Read the model definition and answer for the solid it produces. Units are mm, in the model's axes. A direction names the side the tool comes from. Coordinates: 2 decimals unless noted, no trailing zeros. Loops run counter-clockwise (first coordinate to the right, second up) from the corner with the lowest first, then second, coordinate; pieces in that order, holes last. Notation, with made-up numbers: (43.25, 88) -> (57.25, 88) arc R20 ccw to (57.25, 95) -> close; hole circle Ø8 at (74.25, 23). An arc over 180 degrees is marked (long way). Answer as a JSON object with one key per item and string values. Group by question number.
Q1. Each of these flat-tipped pins is pushed along its axis until it touches: P1, Ø11, axis at x = -0.5, z = -4.5, coming from the -Y side; P2, Ø7, axis at x = 0.5, z = -0.5, coming from the +Y side; P3, Ø2.5, axis at x = 0, z = -7.75, coming from the +Y side; P4, Ø2, axis at x = -8, y = -466.5, coming from the +Z side. Where does it stop, or does it pass through?
Q2. The part is cut by section C-C on y = -466.1. Write down the section's boundary in (x, z) (3 decimals).
Q3. Determine the mould class of faces 4 (the flat face through (3, -468.875, -11)), 5 (the cylindrical face through (-11.64, -466.19, 6.06)), 6 (the flat face through (0, -466.475, 0)) for opening direction Z: released by +Z, released by -Z, zero draft, split by the parting line, or undercut.
Q4. For faces 1 (the cylindrical face through (7.52, -468.38, 8.2)), 2 (the flat face through (-3, -463.275, 3)), 3 (the cylindrical face through (-1.917, -464.853, -2.5)), determine the directions among +Z, -Z, +X, -X, +Y, -Y from which every point of the face is accessible in a straight line to the end or side of a thin tool.
Q5. Straight lines are drawn through the part: line 1 along X through (y, z) = (-468.4, 0) (3 decimals); line 2 along X through (y, z) = (-465.5, 0) (3 decimals); line 3 along Y through (x, z) = (6.75, -8.5). For each, find the intervals that lie inside material, in ascending order. Write a range as [from, to].
Q6. The part is cut by section B-B on z = 0. Write down the section's boundary in (x, y) (3 decimals), and give its area (4 significant figures).
Q7. The part is cut by section A-A on x = 0. Write down the section's boundary in (y, z) (3 decimals).
from build123d import *

# Parameters (mm, degrees)
SKETCH8_R           = 13.125
BOSS_EXTRUDE2_DEPTH = 5.6
SKETCH9_R           = 11.125
CUT_EXTRUDE4_DEPTH  = 1
SKETCH10_R          = 3.15
CUT_EXTRUDE5_DEPTH  = 3.2
CHAMFER2_SIZE       = 0.3
SKETCH11_R          = 1.7
CUT_EXTRUDE6_DEPTH  = 20.38791505


with BuildPart() as part:
    # Sketch8 → Boss-Extrude2 (new body)
    with BuildSketch(Plane(origin=(0, -463.275483874, 0), x_dir=(0.32790942623068436, 0, 0.9447091659283631), z_dir=(0, 1, 0))):
        with Locations(Location((0, 0, 0), (0, 0, 340.858064804))):
            Circle(SKETCH8_R)
    extrude(amount=-BOSS_EXTRUDE2_DEPTH)

    # Sketch9 → Cut-Extrude4 (cut)
    with BuildSketch(Plane(origin=(0, -468.875483874, 0), x_dir=(-1, 0, 0), z_dir=(0, -1, 0))):
        with Locations(Location((0, 0, 0), (0, 0, 90))):
            Circle(SKETCH9_R)
    extrude(amount=-CUT_EXTRUDE4_DEPTH, mode=Mode.SUBTRACT)

    # Sketch10 → Cut-Extrude5 (cut)
    with BuildSketch(Plane(origin=(0, -463.275483874, 0), x_dir=(1, 0, 0), z_dir=(0, 1, 0))):
        with Locations(Location((0, 0, 0), (0, 0, 270))):
            Circle(SKETCH10_R)
    extrude(amount=-CUT_EXTRUDE5_DEPTH, mode=Mode.SUBTRACT)

    # Chamfer2
    chamfer2_edges = [part.edges().sort_by_distance(p)[0] for p in [
        (0, -463.275483874, -13.125),
    ]]
    chamfer(chamfer2_edges, length=CHAMFER2_SIZE)

    # Sketch11 → Cut-Extrude6 (cut, through all)
    with BuildSketch(Plane(origin=(0, -463.275483874, 0), x_dir=(1, 0, 0), z_dir=(0, 1, 0))):
        with Locations(Location((0, -7.75, 0), (0, 0, 270))):
            Circle(SKETCH11_R)
        with Locations(Location((0, 7.75, 0), (0, 0, 270))):
            Circle(SKETCH11_R)
    extrude(amount=-CUT_EXTRUDE6_DEPTH, mode=Mode.SUBTRACT)


solid = part.part
Final values:
{
 "1": {"P1": "stops at y = -467.88", "P2": "stops at y = -463.28", "P3": "passes through", "P4": "stops at z = 11.1"},
 "2": {"outline": "circle Ø26.25 at (0, 0); hole circle Ø6.3 at (0, 0); hole circle Ø3.4 at (0, -7.75); hole circle Ø3.4 at (0, 7.75)"},
 "3": {"face 4": "zero draft", "face 5": "split by the parting line", "face 6": "undercut"},
 "4": {"face 1": "-Y", "face 2": "+Z, -Z, +X, -X, +Y", "face 3": "+Y"},
 "5": {"line 1": "x = [-13.125, -11.125], [11.125, 13.125]", "line 2": "x = [-13.125, -3.15], [3.15, 13.125]", "line 3": "y = [-467.88, -463.28]"},
 "6": {"outline": "(-13.125, -468.875) -> (-11.125, -468.875) -> (-11.125, -467.875) -> (11.125, -467.875) -> (11.125, -468.875) -> (13.125, -468.875) -> (13.125, -463.575) -> (12.825, -463.275) -> (3.15, -463.275) -> (3.15, -466.475) -> (-3.15, -466.475) -> (-3.15, -463.275) -> (-12.825, -463.275) -> (-13.125, -463.575) -> close", "area": "104.5 mm2"},
 "7": {"outline": "(-468.875, -13.125) -> (-463.575, -13.125) -> (-463.275, -12.825) -> (-463.275, -9.45) -> (-467.875, -9.45) -> (-467.875, -11.125) -> (-468.875, -11.125) -> close; (-468.875, 11.125) -> (-467.875, 11.125) -> (-467.875, 9.45) -> (-463.275, 9.45) -> (-463.275, 12.825) -> (-463.575, 13.125) -> (-468.875, 13.125) -> close; (-467.875, -6.05) -> (-463.275, -6.05) -> (-463.275, -3.15) -> (-466.475, -3.15) -> (-466.475, 3.15) -> (-463.275, 3.15) -> (-463.275, 6.05) -> (-467.875, 6.05) -> close"}
}
